Could you check a few things on this drawing? It's one solid part, dimensions in mm from its lowest x, y, z. Coordinates: 2 decimals unless noted, no trailing zeros. Order: outer loops, then holes, each group sorted by start corner. A loop starts at its lowest first (then second) coordinate and runs counter-clockwise, first axis right, second up.
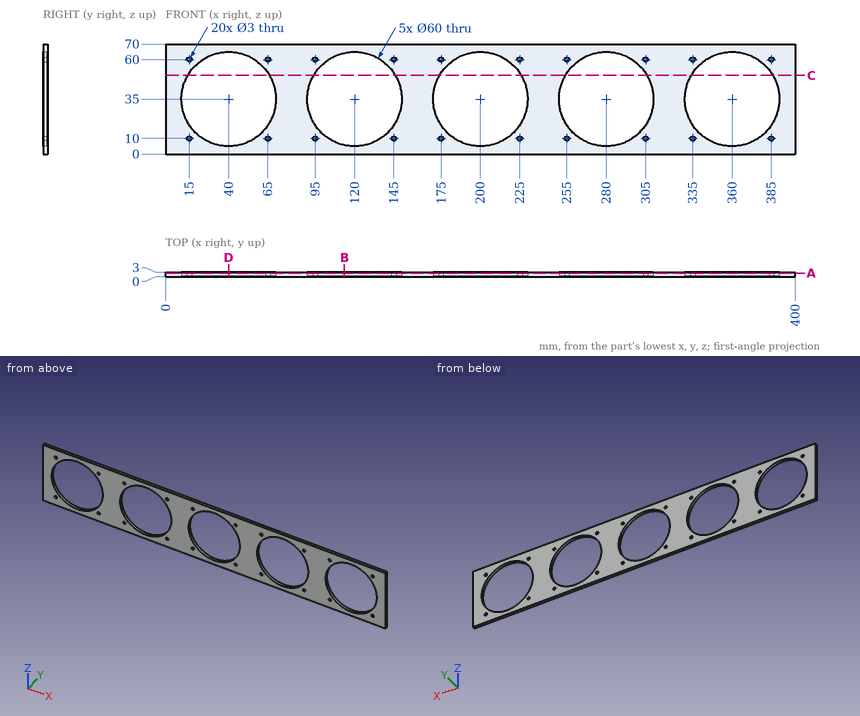
Q1. If we section it at D-D on x = 40: Write out the boundary of the cut face in (y, z).
Q2. I need wall thicknesses on L1, parallel to X at y = 2, z = 35; L2, parallel to X at y = 1.4, z = 33; L3, parallel to Z at x = 202, y = 0.7. Which ranges of each line are inside material? Lowest first, please.
Q3. If we section it at C-C on z = 50: Write out the boundary of the cut face in (x, y).
Q4. If we section it at A-A on y = 2.3: Give the number of separate pieces and of enclosed holes in the cut face, then the cut area to 3 significant figures.
Q5. Will this pin go through, and if not, where does the flat tip stop? pin 1 (8 mm diameter, centred on x = 215, z = 17.5, fed in from +Y).
Q6. If we section it at B-B on x = 113.5: Write out the boundary of the cut face in (y, z).
Reply:
1. outline: (0, 0) - (3, 0) - (3, 5) - (0, 5) - close; (0, 65) - (3, 65) - (3, 70) - (0, 70) - close
2. L1: x = 0 to 10, 70 to 90, 150 to 170, 230 to 250, 310 to 330, 390 to 400
2. L2: x = 0 to 10.07, 69.93 to 90.07, 149.93 to 170.07, 229.93 to 250.07, 309.93 to 330.07, 389.93 to 400
2. L3: z = 0 to 5.07, 64.93 to 70
3. outline: (0, 0) - (14.02, 0) - (14.02, 3) - (0, 3) - close; (65.98, 0) - (94.02, 0) - (94.02, 3) - (65.98, 3) - close; (145.98, 0) - (174.02, 0) - (174.02, 3) - (145.98, 3) - close; (225.98, 0) - (254.02, 0) - (254.02, 3) - (225.98, 3) - close; (305.98, 0) - (334.02, 0) - (334.02, 3) - (305.98, 3) - close; (385.98, 0) - (400, 0) - (400, 3) - (385.98, 3) - close
4. separate pieces: 1
4. enclosed holes: 25
4. area: 13,700 mm2
5. pin 1: passes through
6. outline: (0, 0) - (3, 0) - (3, 5.71) - (0, 5.71) - close; (0, 64.29) - (3, 64.29) - (3, 70) - (0, 70) - close
